Verification items for the finished model (mm, model axes). Face numbers are marked on the shaded views. Give positions to 0.01 mm unless a question says otherwise; leave off trailing zeros. Order: outer loops, then holes, each group sorted by start corner. A loop starts at its lowest first (then second) coordinate and runs counter-clockwise, first axis right, second up.
(1) Sectioned sample at C-C on y = 8.5. Record the cut outline in (x, z) (3 decimals), plus the area to 3 significant figures.
(2) Mould release check, pull along Z, two halves, no side actions. Record for the marked faces 1, 2, 3 and 4: pulls with the +Z half, pulls with the -Z half, needs draft (parallel to the pull), parting line crosses it, or undercut.
(3) Gauge pin test, flat ends, axial feed: pin 1 (1.5 mm diameter, centred on x = 30, z = 37, fed in from -Y); pin 2 (8 mm diameter, centred on y = 31.5, z = 17.5, fed in from -X); pin 3 (8 mm diameter, centred on y = 44.5, z = -8, fed in from +X); pin 4 (5 mm diameter, centred on x = 1, z = 28.5, fed in from +Y). Record the tip position at first contact, or that the pin passes through.
(4) Sectioned sample at A-A on x = 0. Record the cut outline in (y, z) (3 decimals), plus the area to 3 significant figures.
(5) Sectioned sample at B-B on z = 0. Record the cut outline in (x, y) (3 decimals).
(6) Sectioned sample at D-D on y = 39.5. Record the cut outline in (x, z), plus the area to 3 significant figures.
(7) Scan lines: L1, parallel to X at y = 12, z = 0 (3 decimals); L2, parallel to Y at x = -40, z = 28; L3, parallel to Z at x = 11, y = 11.5. Record each from-to range of solid material in increasing order.
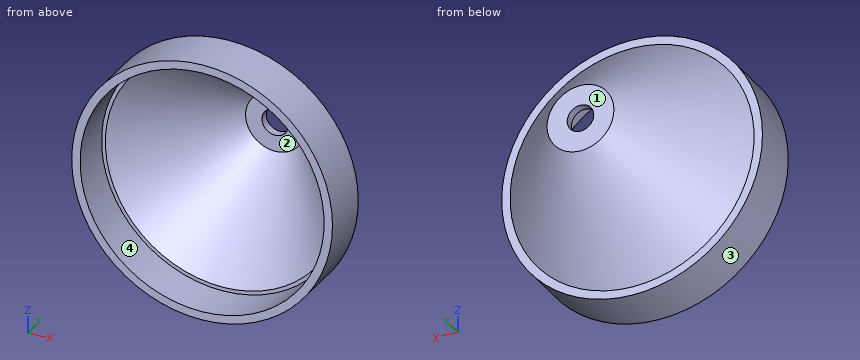
```python
from build123d import *

# Parameters (mm, degrees)
SKETCH1_R                   = 49.53
BOSS_EXTRUDE1_DEPTH         = 76.2
SHELL1_T                    = -3.175
F_3_8_CLEARANCE_HOLE1_D     = 10.0838
F_3_8_CLEARANCE_HOLE1_DEPTH = 25.4
F_3_8_CLEARANCE_HOLE1_TIP   = 3.029479155


with BuildPart() as part:
    # Sketch1 → Boss-Extrude1 (new body)
    with BuildSketch(Plane(origin=(0, 0, 0), x_dir=(1, 0, 0), z_dir=(0, 1, 0))):
        with Locations(Location((0, 0, 0), (0, 0, 90))):
            Circle(SKETCH1_R)
    extrude(amount=BOSS_EXTRUDE1_DEPTH)

    # Sketch8 → Cut-Revolve1 (revolve, cut)
    with BuildSketch(Plane.XY, mode=Mode.PRIVATE) as cut_revolve1_sk:
        Polygon((49.53, 19.05), (46.355, 19.05), (12.7, 57.15), (0, 57.15), (0, 76.2), (49.53, 76.2), align=None)
    revolve(cut_revolve1_sk.sketch.rotate(Axis((0, 76.2, 0), (0, -1, 0)), 270), axis=Axis((0, 76.2, 0), (0, -1, 0)), mode=Mode.SUBTRACT)

    # Shell1
    shell1_openings = [part.faces().sort_by_distance(p)[0] for p in [
        (0, 0, 0),
    ]]
    offset(amount=SHELL1_T, openings=shell1_openings, kind=Kind.INTERSECTION)

    # 3/8 Clearance Hole1
    with Locations(Plane(origin=(0, 57.15, 0), x_dir=(1, 0, 0), z_dir=(0, 1, 0))):
        with Locations((0, 0)):
            Hole(F_3_8_CLEARANCE_HOLE1_D / 2, depth=F_3_8_CLEARANCE_HOLE1_DEPTH)
            with Locations((0, 0, -(F_3_8_CLEARANCE_HOLE1_DEPTH + F_3_8_CLEARANCE_HOLE1_TIP / 2))):  # 118° drill point
                Cone(0, F_3_8_CLEARANCE_HOLE1_D / 2, F_3_8_CLEARANCE_HOLE1_TIP, mode=Mode.SUBTRACT)


solid = part.part
```
Ans:
1. outline: circle Ø99.06 at (0, 0); hole circle Ø92.71 at (0, 0)
1. area: 956 mm2
2. face 1: needs draft
2. face 2: undercut
2. face 3: parting line crosses it
2. face 4: undercut
3. pin 1: stops at y = 0
3. pin 2: stops at x = -35.17
3. pin 3: stops at x = 26.38
3. pin 4: stops at y = 42.07
4. outline: (0, -49.53) - (19.05, -49.53) - (19.05, -46.355) - (57.15, -12.7) - (57.15, -5.042) - (53.975, -5.042) - (53.975, -11.268) - (15.875, -44.923) - (15.875, -46.355) - (0, -46.355) - close; (0, 46.355) - (15.875, 46.355) - (15.875, 44.923) - (53.975, 11.268) - (53.975, 5.042) - (57.15, 5.042) - (57.15, 12.7) - (19.05, 46.355) - (19.05, 49.53) - (0, 49.53) - close
4. area: 492 mm2
5. outline: (-49.53, 0) - (-46.355, 0) - (-46.355, 15.875) - (-44.923, 15.875) - (-11.268, 53.975) - (-5.042, 53.975) - (-5.042, 57.15) - (-12.7, 57.15) - (-46.355, 19.05) - (-49.53, 19.05) - close; (5.042, 53.975) - (11.268, 53.975) - (44.923, 15.875) - (46.355, 15.875) - (46.355, 0) - (49.53, 0) - (49.53, 19.05) - (46.355, 19.05) - (12.7, 57.15) - (5.042, 57.15) - close
6. outline: circle Ø56.58 at (0, 0); hole circle Ø48.11 at (0, 0)
6. area: 697 mm2
7. L1: x = -49.53 to -46.355, 46.355 to 49.53
7. L2: y = 0 to 19.05
7. L3: z = -48.29 to -45.03, 45.03 to 48.29
